```python
from build123d import *

# Parameters (mm, degrees)
EXTRUDE_1_DEPTH   = 2
HOLE_WIZARD_M81_D = 9
CHAMFER_1_SIZE    = 2.5


with BuildPart() as part:
    # Эскиз3 → Бобышка-Вытянуть1 (new body)
    with BuildSketch(Plane(origin=(0, 0, 0), x_dir=(1, 0, 0), z_dir=(0, 0, -1))):
        Polygon((0, 0), (80, 0), (80, 80), (60, 114.641016151), (0, 80), align=None)
    extrude(amount=EXTRUDE_1_DEPTH)

    # Отверстие с зазором M81 (through all)
    with Locations(Plane(origin=(0, 0, -2), x_dir=(1, 0, 0), z_dir=(0, 0, -1))):
        with Locations((20, 20), (60, 20), (17.320508076, 66.905989232), (52.679491924, 87.320508076)):
            Hole(HOLE_WIZARD_M81_D / 2)

    # Фаска1
    chamfer_1_edges = [part.edges().sort_by_distance(p)[0] for p in [
        (60, -114.641016151, -1),
        (80, 0, -1),
        (0, 0, -1),
    ]]
    chamfer(chamfer_1_edges, length=CHAMFER_1_SIZE)


solid = part.part
```
Here's how the part is built. I have some questions about the finished solid (model axes, mm). Coordinates: 2 decimals unless noted, no trailing zeros. Order: outer loops, then holes, each group sorted by start corner. A loop starts at its lowest first (then second) coordinate and runs counter-clockwise, first axis right, second up.
Item 1: I'm going to push flat-ended pins straight in: pin 1 Ø12 at (x, y) = (33, -101.5) entering from +Z; pin 2 Ø8 at (x, y) = (17.32, -66.91) entering from -Z. Where does each tip first touch, or does it pass through?
Response values:
pin 1: stops at z = 0
pin 2: passes through
Item 2: Thinking about a two-plate mould opening in X: for faces 1 (the face through (15.244, -62.914, -0.986)), 2 (the face through (70.756, -96.011, -0.986)), 3 (the face through (39, -45, 0)), 4 (the face through (1.2, -1.3, -1)), which applies, pulls with the +X half, pulls with the -X half, needs draft (parallel to the pull), parting line crosses it, or undercut?
Response values:
face 1: undercut
face 2: pulls with the +X half
face 3: needs draft
face 4: pulls with the -X half
Item 3: I need wall thicknesses on probe 1 along X at (y, z) = (-20, -0.85); probe 2 along X at (y, z) = (-17, -0.7); probe 3 along Y at (x, z) = (20, -0.55). Which ranges of each line are inside material? Lowest first, please.
Response values:
probe 1: x = 0 to 15.5, 24.5 to 55.5, 64.5 to 80
probe 2: x = 0 to 16.65, 23.35 to 56.65, 63.35 to 80
probe 3: y = -91.55 to -70.52, -63.29 to -24.5, -15.5 to 0
Item 4: If we section it at C-C, the plane x = 20: List the corners of the cut face in (y, z) for me, then the cut area to 3 significant figures.
Response values:
outline: (-91.55, -2) - (-70.52, -2) - (-70.52, 0) - (-91.55, 0) - close; (-63.29, -2) - (-24.5, -2) - (-24.5, 0) - (-63.29, 0) - close; (-15.5, -2) - (0, -2) - (0, 0) - (-15.5, 0) - close
area: 151 mm2
Item 5: If we section it at B-B, the plane x = 50.5: List the corners of the cut face in (y, z) for me, then the cut area to 3 significant figures.
Response values:
outline: (-109.16, -2) - (-91.26, -2) - (-91.26, 0) - (-109.16, 0) - close; (-83.38, -2) - (0, -2) - (0, 0) - (-83.38, 0) - close
area: 203 mm2
Item 6: If we section it at A-A, the plane y = -20: List the corners of the cut face in (x, z) for me.
Response values:
outline: (0, -2) - (15.5, -2) - (15.5, 0) - (0, 0) - close; (24.5, -2) - (55.5, -2) - (55.5, 0) - (24.5, 0) - close; (64.5, -2) - (80, -2) - (80, 0) - (64.5, 0) - close
Item 7: If we section it at D-D, the plane z = -0.85: List the corners of the cut face in (x, y) for me.
Response values:
outline: (0, -80) - (57.83, -113.39) - (61.25, -112.48) - (80, -80) - (80, -2.5) - (77.5, 0) - (2.5, 0) - (0, -2.5) - close; hole circle Ø9 at (17.32, -66.91); hole circle Ø9 at (20, -20); hole circle Ø9 at (52.68, -87.32); hole circle Ø9 at (60, -20)
